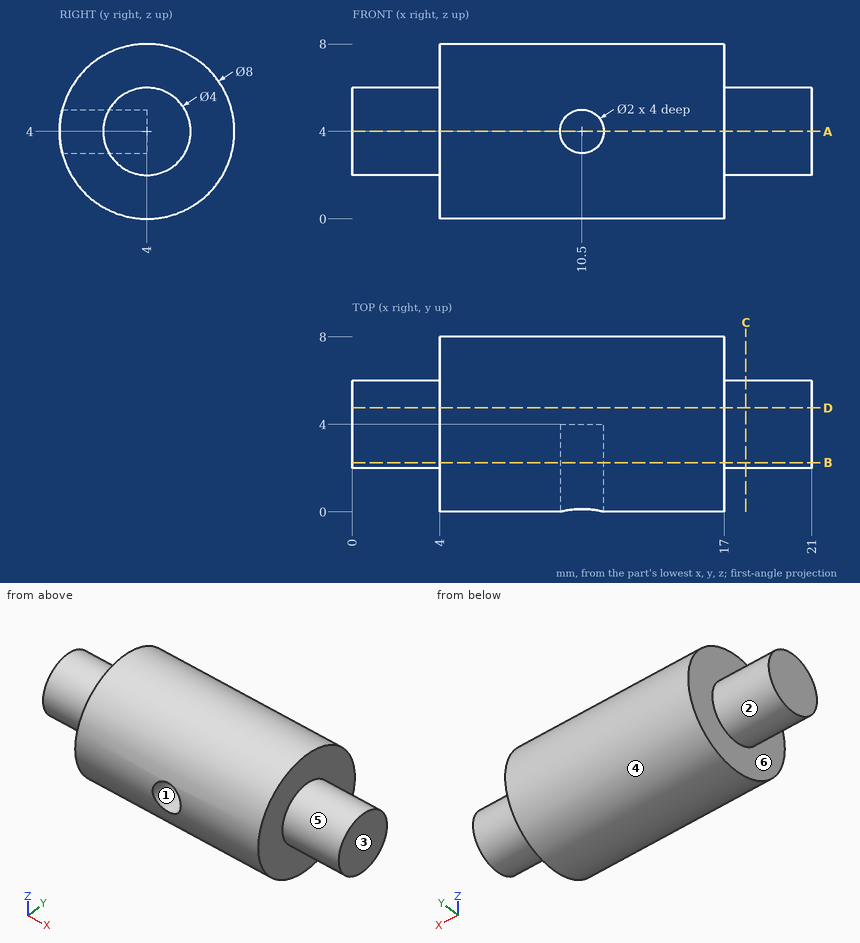
Geometry: see drawing. Coordinates: mm, zero at the bounding-box minimum. A direction names the side the tool comes from. Coordinates: 2 decimals unless noted, no trailing zeros. Order: outer loops, then holes, each group sorted by start corner. A loop starts at its lowest first (then second) coordinate and runs counter-clockwise, first axis right, second up. Notation, with made-up numbers: (10.25, 17.5) - (36.25, 17.5) arc R22 ccw to (36.25, 41.5) - close; hole circle Ø2 at (24, 71). An arc over 180 degrees is marked (long way). Write each question's results on one line, items separated by ' | '.
1) Pin query (flat end, axial travel): pin 1 (0.6 mm diameter, centred on x = 10.5, z = 4, fed in from -Y). Return the tip coordinate at first contact, or that it passes through.
Results list:
pin 1: y = 4
2) Section D-D, the plane y = 4.75. Return loops of the section in (x, z), plus the area to 3 significant figures.
Results list:
outline: (0, 2.15) - (4, 2.15) - (4, 0.07) - (17, 0.07) - (17, 2.15) - (21, 2.15) - (21, 5.85) - (17, 5.85) - (17, 7.93) - (4, 7.93) - (4, 5.85) - (0, 5.85) - close | area: 132 mm^2
3) Line query: line 1 (X direction, y = 7, z = 6.5); line 2 (Z direction, x = 10.5, y = 1.15); line 3 (Z direction, x = 10.5, y = 1.25). Output: solid intervals per line, ascending. Write a range as from..to.
Results list:
line 1: 4..17 | line 2: 1.19..3, 5..6.81 | line 3: 1.1..3, 5..6.9
4) Section C-C, the plane x = 18. Return loops of the section in (y, z).
Results list:
outline: circle Ø4 at (4, 4)
5) Section A-A, the plane z = 4. Return loops of the section in (x, y), plus the area to 3 significant figures.
Results list:
outline: (0, 2) - (4, 2) - (4, 0) - (9.5, 0) - (9.5, 4) - (11.5, 4) - (11.5, 0) - (17, 0) - (17, 2) - (21, 2) - (21, 6) - (17, 6) - (17, 8) - (4, 8) - (4, 6) - (0, 6) - close | area: 128 mm^2
6) Pull-direction query (X, two-part tool) for the marked faces 1, 2 and 3; classes: pulls with the +X half, pulls with the -X half, needs draft (parallel to the pull), parting line crosses it, or undercut.
Results list:
face 1: undercut | face 2: needs draft | face 3: pulls with the +X half
7) Set-up query: the marked faces 4, 5 and 6. Return all of +Z, -Z, +X, -X, +Y, -Y with unobstructed straight access to the full face (end or side cutting, diameter ignored); none if empty.
Results list:
face 4: +X, -X | face 5: +X | face 6: -X
8) Section B-B, the plane y = 2.25. Return loops of the section in (x, z).
Results list:
outline: (0, 3.03) - (4, 3.03) - (4, 0.4) - (17, 0.4) - (17, 3.03) - (21, 3.03) - (21, 4.97) - (17, 4.97) - (17, 7.6) - (4, 7.6) - (4, 4.97) - (0, 4.97) - close; hole circle Ø2 at (10.5, 4)
